```python
from build123d import *

# Parameters (mm, degrees)
MODEL_R             = 0.925
BOSS_EXTRUDE1_DEPTH = 3
FILLET1_R           = 1


with BuildPart() as part:
    # Model → Boss-Extrude1 (new body)
    with BuildSketch(Plane.XY):
        Polygon((142.344747242, 270.871489374), (153.37187249, 271.263447748), (162.091473536, 274.767362889), (160.85900272, 279.367807803), (179.260689602, 284.297666211), (178.028627015, 288.898354165), (208.019481767, 296.93522173), (209.252454514, 292.334187025), (227.65276755, 297.263677376), (230.276744897, 287.46915479), (275.445873116, 299.572514112), (298.39980436, 213.909597233), (260.87259576, 203.855963236), (255.943287021, 222.255598366), (248.650938057, 220.301667543), (251.115775513, 211.101166572), (220.422247557, 202.878292884), (219.189771603, 207.477473721), (213.081966369, 205.841177268), (214.314693354, 201.241059665), (196.039346948, 196.343682115), (196.007810089, 177.840578221), (186.702312667, 152.27893851), (161.565977706, 161.426447529), (132.435827139, 161.934428279), (107.399642776, 152.824765622), (97.980730454, 178.710864183), (99.858189105, 195.997881416), (81.758593313, 200.846808858), (82.991121062, 205.447466285), (76.882860045, 207.083884844), (75.650856625, 202.485184579), (44.956891994, 210.708175253), (47.421773629, 219.90863481), (40.129543563, 221.862285479), (35.199939127, 203.463086712), (-2.32684459, 213.517448416), (20.785545351, 299.774827661), (65.955825932, 287.671594898), (68.42160019, 296.872525865), (86.820985153, 291.940533454), (88.054439652, 296.542595671), (118.044472643, 288.503706576), (116.812112756, 283.905728394), (135.211333861, 278.973779905), (133.979081507, 274.376202933), align=None)
        with Locations((23.035554, 295.877718337)):
            Circle(MODEL_R, mode=Mode.SUBTRACT)
        with Locations((109.301822433, 156.902965293)):
            Circle(MODEL_R, mode=Mode.SUBTRACT)
        with Locations((184.800560745, 156.35733766)):
            Circle(MODEL_R, mode=Mode.SUBTRACT)
        with Locations((193.847437398, 289.84318413)):
            Circle(MODEL_R, mode=Mode.SUBTRACT)
        with Locations((102.225689846, 289.449650012)):
            Circle(MODEL_R, mode=Mode.SUBTRACT)
        with Locations((273.195899511, 295.675384555)):
            Circle(MODEL_R, mode=Mode.SUBTRACT)
        with Locations((1.570241786, 215.767496811)):
            Circle(MODEL_R, mode=Mode.SUBTRACT)
        with Locations((294.502731407, 216.159668876)):
            Circle(MODEL_R, mode=Mode.SUBTRACT)
        with Locations((80.760413887, 209.339268578)):
            Circle(MODEL_R, mode=Mode.SUBTRACT)
        with Locations((215.312231294, 209.732861073)):
            Circle(MODEL_R, mode=Mode.SUBTRACT)
        with Locations((133.281102646, 207.339464548)):
            Circle(MODEL_R, mode=Mode.SUBTRACT)
        with Locations((162.46850521, 207.598897954)):
            Circle(MODEL_R, mode=Mode.SUBTRACT)
        with Locations((142.522359716, 244.531276159)):
            Circle(MODEL_R, mode=Mode.SUBTRACT)
        with Locations((153.549484965, 244.723703681)):
            Circle(MODEL_R, mode=Mode.SUBTRACT)
    extrude(amount=BOSS_EXTRUDE1_DEPTH)

    # Fillet1
    fillet1_edges = [part.edges().sort_by_distance(p)[0] for p in [
        (-2.32684459, 213.517448416, 1.5),
        (20.785545351, 299.774827661, 1.5),
        (68.42160019, 296.872525865, 1.5),
        (88.054439652, 296.542595671, 1.5),
        (118.044472643, 288.503706576, 1.5),
        (135.211333861, 278.973779905, 1.5),
        (160.85900272, 279.367807803, 1.5),
        (178.028627015, 288.898354165, 1.5),
        (208.019481767, 296.93522173, 1.5),
        (227.65276755, 297.263677376, 1.5),
        (275.445873116, 299.572514112, 1.5),
        (298.39980436, 213.909597233, 1.5),
        (260.87259576, 203.855963236, 1.5),
        (251.115775513, 211.101166572, 1.5),
        (220.422247557, 202.878292884, 1.5),
        (214.314693354, 201.241059665, 1.5),
        (186.702312667, 152.27893851, 1.5),
        (107.399642776, 152.824765622, 1.5),
        (81.758593313, 200.846808858, 1.5),
        (75.650856625, 202.485184579, 1.5),
        (44.956891994, 210.708175253, 1.5),
        (35.199939127, 203.463086712, 1.5),
    ]]
    fillet(fillet1_edges, radius=FILLET1_R)


solid = part.part
```
Can you work these out from the model? Positions are in its coordinate system, mm. A direction names the side the tool comes from. Coordinates: 2 decimals unless noted, no trailing zeros. Order: outer loops, then holes, each group sorted by start corner. A loop starts at its lowest first (then second) coordinate and runs counter-clockwise, first axis right, second up. Notation, with made-up numbers: (-32.75, 88.5) - (-5.75, 88.5) arc R27 cw to (-5.75, 114.5) - close; hole circle Ø4 at (-39, 18.25). An arc over 180 degrees is marked (long way). Answer in a Markdown table with one row per item.
1. Suppose I cut it at A-A (y = 266.5). Please give me the cut outline in (x, z).
Reply:
| item | result |
|---|---|
| outline | (11.87, 0) - (284.31, 0) - (284.31, 3) - (11.87, 3) - close |
2. Suppose I cut it at C-C (x = 173). Please give me the cut outline in (y, z).
Reply:
| item | result |
|---|---|
| outline | (157.27, 0) - (282.62, 0) - (282.62, 3) - (157.27, 3) - close |
3. Suppose I cut it at B-B (z = 0.45). Give the number of separate pieces and of enclosed holes in the cut face, and give its area (3 significant figures).
Reply:
| item | result |
|---|---|
| separate pieces | 1 |
| enclosed holes | 14 |
| area | 27,800 mm^2 |
4. For pin 1 (3 mm diameter, centred on x = 294.5, y = 216.16, fed in from -Z); pin 2 (1.1 mm diameter, centred on x = 193.85, y = 289.84, fed in from -Z); pin 3 (1 mm diameter, centred on y = 189.5, z = 1, fed in from +X), each with a flat end and sliding along its axis, tell me the tip position at first contact or that it passes through.
Reply:
| item | result |
|---|---|
| pin 1 | stops at z = 0 |
| pin 2 | passes through |
| pin 3 | stops at x = 196.03 |
5. If I drill on line 1 along X through (y, z) = (244.5, 2); line 2 along X through (y, z) = (276.5, 2.1); line 3 along Y through (x, z) = (69.5, 0.45), over which ranges is the centre line in solid material (lowest first)?
Reply:
| item | result |
|---|---|
| line 1 | x = 5.97 to 141.6, 143.45 to 152.65, 154.45 to 290.2 |
| line 2 | x = 14.55 to 134.55, 161.63 to 281.63 |
| line 3 | y = 204.13 to 296.58 |
6. If we mould it in two halves opening along Z, with no side actions, what happens to faces 4 (the flat face through (192.828, 292.864, 1.479)), 5 (the flat face through (150, 227, 0)), 6 (the flat face through (150, 227, 3))? For each: pulls with the +Z half, pulls with the -Z half, needs draft (parallel to the pull), parting line crosses it, or undercut.
Reply:
| item | result |
|---|---|
| face 4 | needs draft |
| face 5 | pulls with the -Z half |
| face 6 | pulls with the +Z half |
7. For faces 1 (the flat face through (102.583, 166.063, 1.479)), 2 (the flat face through (235.97, 207.044, 1.479)), 3 (the flat face through (43.544, 293.677, 1.479)), which set-ups out of +Z, -Z, +X, -X, +Y, -Y let a thin tool reach every point of the face, with its end or its side?
Reply:
| item | result |
|---|---|
| face 1 | +Z, -Z, -X, -Y |
| face 2 | +Z, -Z, -Y |
| face 3 | +Z, -Z, +Y |
